Input: dimensioned drawing with shaded views. Units: mm. Origin: part minimum x, y, z. A direction names the side the tool comes from. Coordinates: 2 decimals unless noted, no trailing zeros. Order: outer loops, then holes, each group sorted by start corner. A loop starts at its lowest first (then second) coordinate and runs counter-clockwise, first axis right, second up.
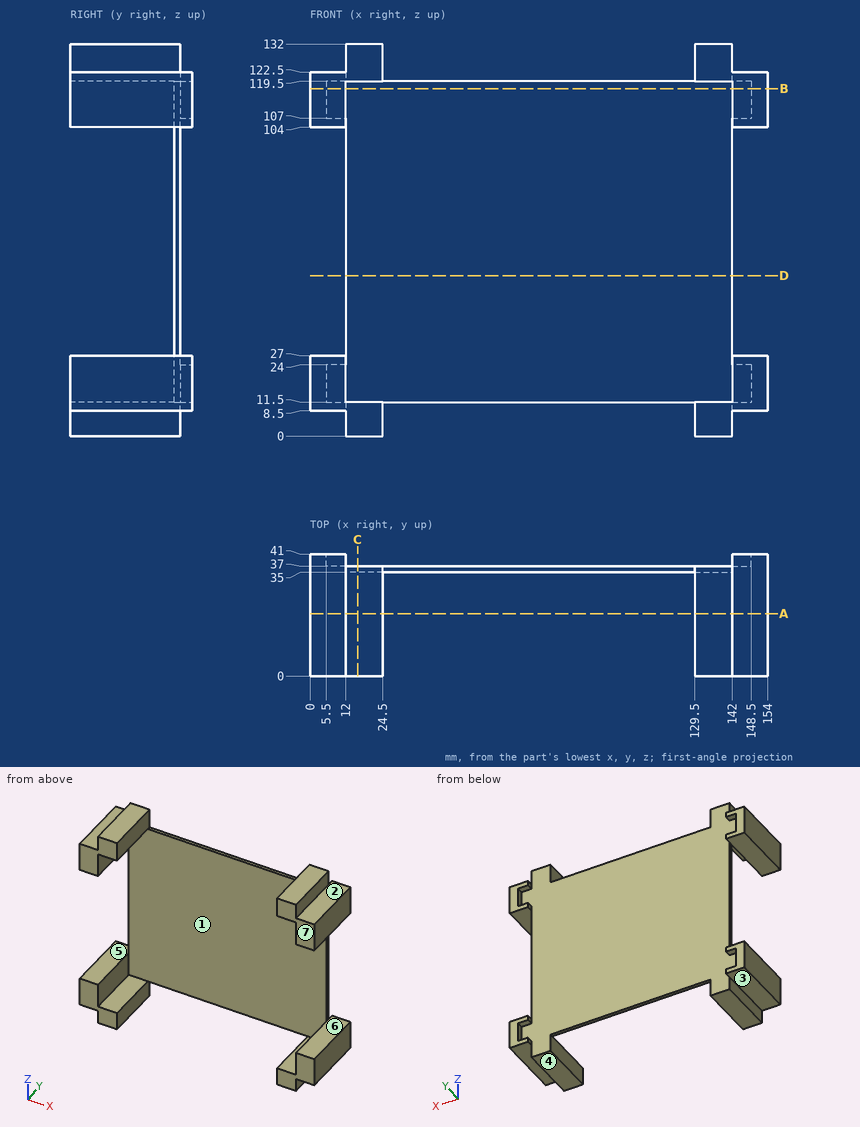
1. Material intervals for line 1 along Z through (x, y) = (19, 25.5); line 2 along X through (y, z) = (23.5, 6.5); line 3 along X through (y, z) = (10, 119), sorted ascending.
2. Section query A-A, the plane y = 21. Count the separate pieces of the cut face and the enclosed holes in it, plus the area to 3 significant figures.
3. Access query for the marked faces 1, 2 and 3. Directions: +Z, -Z, +X, -X, +Y, -Y. A direction counts if a zero-diameter tool reaches every point of the face in a straight line with its end or side. Return the directions, or none.
4. Contact query for flat-ended pins moving along their axis: P1, Ø1, axis at x = 71, z = 104, coming from the -Y side; P2, Ø1.2, axis at x = 9, y = 38.5, coming from the -Z side; P3, Ø2.5, axis at y = 19, z = 3.5, coming from the +X side; P4, Ø3, axis at x = 105, y = 32.5, coming from the -Z side. Output: stop coordinate, or through.
5. Draft query along Z for the marked faces 4, 5, 6 and 7. Return one class per face: +Z half, -Z half, draft (parallel to the pull), parting line (faces both ways), or undercut.
6. Section query C-C, the plane x = 16. Output: boundary loops of the cut face in (y, z).
7. Section query D-D, the plane z = 54. Output: boundary loops of the cut face in (x, y), plus the area to 3 significant figures.
8. Section query B-B, the plane z = 117. Output: boundary loops of the cut face in (x, y).
Answer key:
1. line 1: z = 0 to 11.5, 119.5 to 132
1. line 2: x = 12 to 24.5, 129.5 to 142
1. line 3: x = 0 to 12, 142 to 154
2. separate pieces: 4
2. enclosed holes: 0
2. area: 1,490 mm2
3. face 1: -Y
3. face 2: +Z, +X, +Y, -Y
3. face 3: -Z, -X, +Y, -Y
4. P1: stops at y = 35
4. P2: stops at z = 8.5
4. P3: stops at x = 142
4. P4: passes through
5. face 4: -Z half
5. face 5: undercut
5. face 6: undercut
5. face 7: draft
6. outline: (0, 0) - (37, 0) - (37, 132) - (0, 132) - (0, 119.5) - (35, 119.5) - (35, 11.5) - (0, 11.5) - close
7. outline: (12, 35) - (142, 35) - (142, 37) - (12, 37) - close
7. area: 260 mm2
8. outline: (0, 0) - (12, 0) - (12, 35) - (142, 35) - (142, 0) - (154, 0) - (154, 41) - (148.5, 41) - (148.5, 37) - (5.5, 37) - (5.5, 41) - (0, 41) - close
